```python
from build123d import *

# Parameters (mm, degrees)
BOSS_EXTRUDE1_DEPTH = 78
SKETCH4_W           = 4
SKETCH4_H           = 5
BOSS_EXTRUDE2_DEPTH = 13
SKETCH5_W           = 4
SKETCH5_H           = 5
BOSS_EXTRUDE3_DEPTH = 13
BOSS_EXTRUDE6_DEPTH = 60


with BuildPart() as part:
    # Sketch2 → Boss-Extrude1 (new body)
    with BuildSketch(Plane(origin=(0, 0, 0), x_dir=(1, 0, 0), z_dir=(0, 1, 0))):
        Polygon((0, 0), (0, -15), (-5, -15), (-5, -2), (-9, -2), (-9, -15), (-14, -15), (-14, 5.798989873), align=None)
    boss_extrude1 = extrude(amount=BOSS_EXTRUDE1_DEPTH)

    # Mirror1: Boss-Extrude1 across plane
    add(boss_extrude1.mirror(Plane(origin=(0, 78, 0), x_dir=(0.9238795325112891, 0, 0.382683432365084), z_dir=(-0.382683432365084, 0, 0.9238795325112892))))

    # Sketch4 → Boss-Extrude2 (add)
    with BuildSketch(Plane(origin=(1.414213562, 0, -1.414213562), x_dir=(-0.7071067811865562, 0, -0.7071067811865389), z_dir=(0.7071067811865389, 0, -0.7071067811865562))):
        with Locations((7, 2.5)):
            Rectangle(SKETCH4_W, SKETCH4_H)
    extrude(amount=BOSS_EXTRUDE2_DEPTH)

    # Sketch5 → Boss-Extrude3 (add)
    with BuildSketch(Plane.XY.offset(2)):
        with Locations((-7, 2.5)):
            Rectangle(SKETCH5_W, SKETCH5_H)
    extrude(amount=BOSS_EXTRUDE3_DEPTH)

    # Sketch14 → Boss-Extrude6 (add)
    with BuildSketch(Plane.XY.offset(15)):
        Polygon((-14, 0), (0, 0), (0, 18), (-5, 18), (-5, 5), (-9, 5), (-9, 18), (-14, 18), align=None)
    boss_extrude6 = extrude(amount=BOSS_EXTRUDE6_DEPTH)

    # Mirror2: Boss-Extrude6 across plane
    add(boss_extrude6.mirror(Plane(origin=(0, 0, 0), x_dir=(0.9238795325112891, 0, 0.3826834323650842), z_dir=(-0.3826834323650841, 0, 0.9238795325112892))))


solid = part.part
```
Input: part model. Units: mm. Frame: model coordinates. A direction names the side the tool comes from. Coordinates: 2 decimals unless noted, no trailing zeros. Write each loop counter-clockwise with the first axis right and the second up, starting at its lowest first coordinate (ties: lowest second). Pieces come first, ordered by that corner, then holes. Notation, with made-up numbers: (42, -8.5) -> (50, -8.5) arc R25 ccw to (50, 16.5) -> close; hole circle Ø2 at (-8.75, 38). An arc over 180 degrees is marked (long way). Answer as a JSON object with one key per item and string values.
1. Mould query, pull axis X, two halves, no side actions, for faces 4 (the face through (50.214, 9.126, -55.852)), 5 (the face through (30, 18, -33)), 6 (the face through (-9, 17, 22)), 7 (the face through (1.5, 13.5, -21.3)). Classes: released by +X, released by -X, zero draft, split by the parting line, or undercut.
Result set:
{"face 4": "released by +X", "face 5": "zero draft", "face 6": "undercut", "face 7": "released by -X"}
2. Material intervals for line 1 (Y direction, x = -8.5, z = 40.5); line 2 (X direction, y = 29, z = 1.5); line 3 (Y direction, x = 30, z = -31.5), sorted ascending. Write a range as from..to.
Result set:
{"line 1": "y = 0..5", "line 2": "x = -14..0", "line 3": "y = 0..18"}
3. Section C-C on x = 29. Return the cut outline in (y, z), then the cut area to 3 significant figures.
Result set:
{"outline": "(0, -48.8) -> (18, -48.8) -> (18, -41.73) -> (5, -41.73) -> (5, -36.07) -> (18, -36.07) -> (18, -29) -> (0, -29) -> close", "area": "283 mm2"}
4. First-contact query: P1, Ø1.5, axis at x = -11.5, z = 59, coming from the +Y side; P2, Ø5, axis at x = 11, y = 36, coming from the -Z side; P3, Ø3, axis at x = -8, y = 50.5, coming from the +Z side. Flat tips, straight axial feed; report the tip coordinate or a pass-through.
Result set:
{"P1": "stops at y = 18", "P2": "stops at z = -12.71", "P3": "stops at z = 15"}
5. Section B-B on y = 57.5. Return the cut outline in (x, z), then the cut area to 3 significant figures.
Result set:
{"outline": "(-14, -5.8) -> (0.71, -20.51) -> (4.24, -16.97) -> (-4.95, -7.78) -> (-2.12, -4.95) -> (7.07, -14.14) -> (10.61, -10.61) -> (0, 0) -> (0, 15) -> (-5, 15) -> (-5, 2) -> (-9, 2) -> (-9, 15) -> (-14, 15) -> close", "area": "397 mm2"}
6. Section A-A on z = 21.5. Return the cut outline in (x, y).
Result set:
{"outline": "(-14, 0) -> (0, 0) -> (0, 18) -> (-5, 18) -> (-5, 5) -> (-9, 5) -> (-9, 18) -> (-14, 18) -> close"}
7. Access query for faces 1 (the face through (9.03, 16.66, -21.76)), 2 (the face through (2.5, 48.42, -18.714)), 3 (the face through (-7, 41, 2)). Directions: +Z, -Z, +X, -X, +Y, -Y. A direction counts if a zero-diameter tool reaches every point of the face in a straight line with its end or side. Return the directions, or none.
Result set:
{"face 1": "+Y", "face 2": "-Z, +X, +Y", "face 3": "+Z, +Y"}
